For this review, take the finished solid that the model builds, in its own axes (mm). Face numbers are marked on the shaded views. Coordinates: 2 decimals unless noted, no trailing zeros. Loops run counter-clockwise (first coordinate to the right, second up) from the corner with the lowest first, then second, coordinate; pieces in that order, holes last. Notation, with made-up numbers: (-20, 74.5) -> (-3, 74.5) arc R25 ccw to (-3, 87.5) -> close; hole circle Ø4 at (49.5, -8.75). An arc over 180 degrees is marked (long way). Use a Markdown table: item, result.
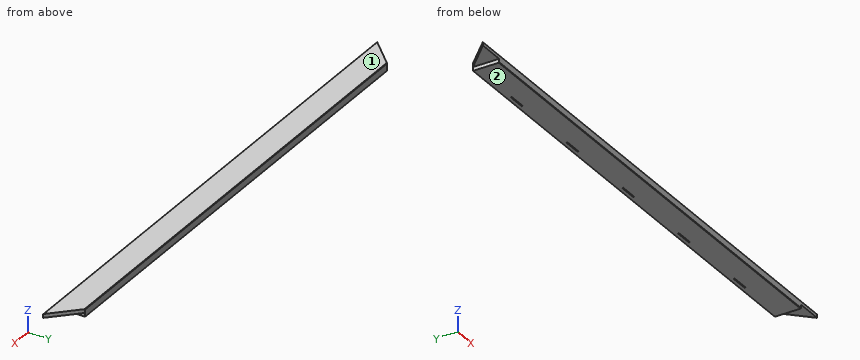
Autodesk Fusion 360 part; units mm, degrees
sketch "Sketch1" plane through (0, 0, 0) normal (0, 0, 1) x (1, 0, 0)
  line L0 (914.4, 44.45) -> (914.4, -44.45) construction
  line L1 (914.4, -44.45) -> (-914.4, -44.45)
  line L2 (-914.4, -44.45) -> (-914.4, 44.45) construction
  line L3 (-914.4, 44.45) -> (914.4, -44.45) construction
  line L4 (914.4, 44.45) -> (-914.4, -44.45) construction
  line L5 (-914.4, -44.45) -> (-825.5, 44.45)
  line L6 (914.4, -44.45) -> (825.5, 44.45)
  line L7 (-914.4, 44.45) -> (-825.5, 44.45) construction
  line L8 (825.5, 44.45) -> (914.4, 44.45) construction
  line L9 (-825.5, 44.45) -> (825.5, 44.45)
  line L10 (0, 0) -> (0, -44.45) construction
  dimension "d27" = 1828.8
  dimension "d40" = 45
  dimension "d41" = 45
  dimension "d42" = 88.9
extrude "Extrude1" add sketch "Sketch1" along normal blind 25.4
sketch "Sketch9" plane through (0, 0, 0) normal (0, 0, 1) x (-1, 0, 0)
  line L0 (825.5, -44.45) -> (914.4, 44.45)
  line L1 (914.4, 44.45) -> (-914.4, 44.45)
  line L2 (-914.4, 44.45) -> (-825.5, -44.45)
  line L3 (914.4, 44.45) -> (825.5, -44.45)
  line L4 (825.5, -44.45) -> (825.5, 44.45)
  line L5 (825.5, 44.45) -> (914.4, 44.45)
  line L6 (-825.5, -44.45) -> (-914.4, 44.45)
  line L7 (-825.5, -44.45) -> (-825.5, 44.45)
  line L8 (-825.5, 44.45) -> (-914.4, 44.45)
  line L9 (-825.5, -44.45) -> (825.5, -44.45)
  line L10 (-825.5, -44.45) -> (-914.4, 44.45)
  line L11 (-914.4, 44.45) -> (914.4, 44.45)
  line L12 (914.4, 44.45) -> (825.5, -44.45)
  line L13 (825.5, -44.45) -> (-825.5, -44.45)
extrude "Extrude8" cut sketch "Sketch9" along normal blind 12.7 contours L0 L1 L3 L4 L5 L11 L12 | L1 L2 L6 L7 L8 L10 L11
chamfer "Chamfer2" distance 1.5875 angle 45 5 edges at (0, -44.45, 25.4) (0, -44.45, 0) (0, 44.45, 25.4) (914.4, -44.45, 19.05) (-914.4, -44.45, 19.05)
sketch "Sketch11" plane through (0, 44.45, 0) normal (0, 1, 0) x (-1, 0, 0)
  line L0 (825.5, 23.8125) -> (-825.5, 23.8125)
  line L1 (-825.5, 23.8125) -> (-825.5, 12.7)
  line L2 (-825.5, 12.7) -> (-825.5, 0)
  line L3 (-825.5, 0) -> (825.5, 0)
  line L4 (825.5, 0) -> (825.5, 12.7)
  line L5 (825.5, 12.7) -> (825.5, 23.8125)
  line L6 (0, 0) -> (30.1625, 0)
  line L7 (0, 0) -> (-30.1625, 0)
  line L8 (0, 0) -> (0, 12.7) construction
  arc A0 (30.1625, 0) -> (-30.1625, 0) centre (0, -29.468) ccw
  line L9 (-609.6, 0) -> (-609.6, 12.7) construction
  line L10 (-609.6, 0) -> (-579.4375, 0)
  line L11 (-609.6, 0) -> (-639.7625, 0)
  arc A1 (-579.4375, 0) -> (-639.7625, 0) centre (-609.6, -29.468) ccw
  line L12 (-304.8, 0) -> (-304.8, 12.7) construction
  line L13 (-304.8, 0) -> (-274.6375, 0)
  line L14 (-304.8, 0) -> (-334.9625, 0)
  arc A2 (-274.6375, 0) -> (-334.9625, 0) centre (-304.8, -29.468) ccw
  line L15 (304.8, 0) -> (304.8, 12.7) construction
  line L16 (304.8, 0) -> (334.9625, 0)
  line L17 (304.8, 0) -> (274.6375, 0)
  arc A3 (334.9625, 0) -> (274.6375, 0) centre (304.8, -29.468) ccw
  line L18 (609.6, 0) -> (609.6, 12.7) construction
  line L19 (609.6, 0) -> (639.7625, 0)
  line L20 (609.6, 0) -> (579.4375, 0)
  arc A4 (639.7625, 0) -> (579.4375, 0) centre (609.6, -29.468) ccw
  point P0 (-609.6, 0)
  point P1 (-304.8, 0)
  point P2 (304.8, 0)
  point P3 (609.6, 0)
  dimension "d59" = 60.325
  dimension "d60" = 12.7
  dimension "d63" = 304.8
  dimension "d64" = 0
extrude "Extrude10" cut sketch "Sketch11" against normal blind 3.7703 from surface at -12.7 contours L3 L19 L20 A4 | L3 L10 L11 A1 | L3 L16 L17 A3 | L3 L13 L14 A2 | L3 L6 L7 A0
equation "d59 = 2 in + ( 3 / 8 ) * 1 in"
equation "d66 = ( -19 / 128 ) * 1 in"
(1) Take a section at C-C on x = -613.5. Write out the cut boundary in (y, z).
Found:
| item | result |
|---|---|
| outline | (-44.45, 1.59) -> (-42.86, 0) -> (27.98, 0) -> (27.98, 12.52) -> (31.75, 12.52) -> (31.75, 0) -> (44.45, 0) -> (44.45, 23.81) -> (42.86, 25.4) -> (-42.86, 25.4) -> (-44.45, 23.81) -> close |
(2) For line 1 along X through (y, z) = (31.5, 4.75); line 2 along X through (y, z) = (-14.5, 12); line 3 along X through (y, z) = (-18.5, 23), list the stretches that pass through material, from the lowest coordinate up.
Found:
| item | result |
|---|---|
| line 1 | x = -825.5 to -634.24, -584.96 to -329.44, -280.16 to -24.64, 24.64 to 280.16, 329.44 to 584.96, 634.24 to 825.5 |
| line 2 | x = -825.5 to 825.5 |
| line 3 | x = -888.45 to 888.45 |
(3) Mouldability with a two-part tool opening along Z and no side actions: class the marked faces 1 and 2 as pulls with the +Z half, pulls with the -Z half, needs draft (parallel to the pull), parting line crosses it, or undercut.
Found:
| item | result |
|---|---|
| face 1 | pulls with the +Z half |
| face 2 | pulls with the -Z half |
(4) Take a section at B-B on z = 17.25. Write out the cut boundary in (x, y), plus the area to 3 significant figures.
Found:
| item | result |
|---|---|
| outline | (-913.28, -43.33) -> (-912.81, -44.45) -> (912.81, -44.45) -> (913.28, -43.33) -> (825.5, 44.45) -> (-825.5, 44.45) -> close |
| area | 155,000 mm^2 |
(5) For pin 1 Ø14 at (y, z) = (20, 3.5) entering from +X; pin 2 Ø10 at (y, z) = (-18.5, 16) entering from +X; pin 3 Ø4 at (y, z) = (-10.5, 5.5) entering from -X, all flat-tipped, find the tip position at first contact; note any pin that passes through.
Found:
| item | result |
|---|---|
| pin 1 | stops at x = 825.5 |
| pin 2 | stops at x = 893.45 |
| pin 3 | stops at x = -825.5 |
(6) Take a section at A-A on y = -14. Write out the cut boundary in (x, z), plus the area to 3 significant figures.
Found:
| item | result |
|---|---|
| outline | (-883.95, 12.7) -> (-825.5, 12.7) -> (-825.5, 0) -> (825.5, 0) -> (825.5, 12.7) -> (883.95, 12.7) -> (883.95, 25.4) -> (-883.95, 25.4) -> close |
| area | 43,400 mm^2 |
(7) Take a section at D-D on x = -290. Write out the cut boundary in (y, z).
Found:
| item | result |
|---|---|
| outline | (-44.45, 1.59) -> (-42.86, 0) -> (27.98, 0) -> (27.98, 10.02) -> (31.75, 10.02) -> (31.75, 0) -> (44.45, 0) -> (44.45, 23.81) -> (42.86, 25.4) -> (-42.86, 25.4) -> (-44.45, 23.81) -> close |
